Input: part model. Units: mm. Frame: model coordinates. Coordinates: 2 decimals unless noted, no trailing zeros. Loops run counter-clockwise (first coordinate to the right, second up) from the corner with the lowest first, then second, coordinate; pieces in that order, holes last.
Item 1: Ray query, line 1 along X through (y, z) = (-72, 0.6); line 2 along Y through (x, z) = (-85, 2.3); line 3 along Y through (x, z) = (0, 1.45). Return the intervals inside material, ascending.
Item 2: Section A-A on y = 59. Return loops of the section in (x, z), and give its area (3 significant figures).
Item 3: Contact query for flat-ended pins moving along their axis: P1, Ø4, axis at x = 50.5, y = -29.5, coming from the -Z side; P2, Ø1.5, axis at x = 92, z = 1.5, coming from the -Y side; P3, Ø2, axis at x = 85, y = -72, coming from the +Z side; P4, Ø1.5, axis at y = -106, z = 1.5, coming from the -X side. Output: stop coordinate, or through.
Item 4: Section B-B on z = 1.2. Give the number of separate pieces and of enclosed holes in the cut face, and give its area (3 significant figures).
Item 5: Pull-direction query (Y, two-part tool) for faces 1 (the cylindrical face through (-1.301, 53.143, 1.521)), 2 (the flat face through (-1, 2, 3)); classes: released by +Y, released by -Y, zero draft, split by the parting line, or undercut.
Autodesk Fusion 360 part; units mm, degrees
sketch "Sketch1" plane through (0, 0, 0) normal (0, 0, 1) x (1, 0, 0)
  line L0 (100, 125) -> (-100, 125)
  line L1 (-100, 125) -> (-100, -125)
  line L2 (-100, -125) -> (100, -125)
  line L3 (100, -125) -> (100, 125)
  line L4 (100, 125) -> (-100, -125) construction
  line L5 (-100, 125) -> (100, -125) construction
  line L6 (-100, 125) -> (100, 125)
  line L7 (100, 125) -> (100, 129)
  line L8 (100, 129) -> (-100, 129)
  line L9 (-100, 129) -> (-100, 125)
  line L10 (-100, -125) -> (100, -125)
  line L11 (100, -125) -> (100, -129)
  line L12 (100, -129) -> (-100, -129)
  line L13 (-100, -129) -> (-100, -125)
  line L14 (100, 125) -> (104, 125)
  line L15 (104, 125) -> (104, -125)
  line L16 (104, -125) -> (100, -125)
  line L17 (100, -125) -> (100, 125)
  line L18 (-100, 125) -> (-104, 125)
  line L19 (-104, 125) -> (-104, -125)
  line L20 (-104, -125) -> (-100, -125)
  line L21 (-100, -125) -> (-100, 125)
  line L22 (-80, -53.8) -> (-80, 2.2) construction
  circle A0 centre (-80, -53.8) radius 1.65 construction
  circle A1 centre (-80, 2.2) radius 1.65 construction
  line L23 (-61.0622, -1) -> (-98.9378, -1) construction
  line L24 (-98.9378, -1) -> (-98.9378, -50.6) construction
  line L25 (-98.9378, -50.6) -> (-61.0622, -50.6) construction
  line L26 (-61.0622, -50.6) -> (-61.0622, -1) construction
  line L27 (-61.0622, -1) -> (-98.9378, -50.6) construction
  line L28 (-98.9378, -1) -> (-61.0622, -50.6) construction
  line L29 (-30.5, 49.5) -> (98.5, 49.5) construction
  line L30 (98.5, 49.5) -> (98.5, -47.5) construction
  line L31 (98.5, -47.5) -> (-30.5, -47.5) construction
  line L32 (-30.5, -47.5) -> (-30.5, 49.5) construction
  circle A2 centre (-28, 43) radius 1.65
  circle A3 centre (94, -42) radius 1.65
  line L33 (-100, 125) -> (-85.5, 125)
  line L34 (-85.5, 125) -> (-85.5, 116)
  line L35 (-85.5, 116) -> (-100, 116)
  line L36 (-100, 116) -> (-100, 125)
  line L37 (100, 125) -> (85.5, 125)
  line L38 (85.5, 125) -> (85.5, 116)
  line L39 (85.5, 116) -> (100, 116)
  line L40 (100, 116) -> (100, 125)
  line L41 (-100, -125) -> (-85.5, -125)
  line L42 (-85.5, -125) -> (-85.5, -116)
  line L43 (-85.5, -116) -> (-100, -116)
  line L44 (-100, -116) -> (-100, -125)
  line L45 (100, -125) -> (85.5, -125)
  line L46 (85.5, -125) -> (85.5, -116)
  line L47 (85.5, -116) -> (100, -116)
  line L48 (100, -116) -> (100, -125)
  line L49 (-100, 100) -> (-104, 100)
  line L50 (100, 100) -> (104, 100)
  line L51 (-100, -100) -> (-104, -100)
  line L52 (100, -100) -> (104, -100)
  line L53 (-85.5, 125) -> (-85.5, 129)
  line L54 (85.5, 125) -> (85.5, 129)
  line L55 (-85.5, -125) -> (-85.5, -129)
  line L56 (85.5, -125) -> (85.5, -129)
  line L57 (-115, -140) -> (-75, -140) construction
  line L58 (-75, -140) -> (-75, -87) construction
  line L59 (-75, -87) -> (-115, -87) construction
  line L60 (-115, -87) -> (-115, -140) construction
  line L61 (-63.3606, -140) -> (-21.3606, -140) construction
  line L62 (-21.3606, -140) -> (-21.3606, -53.8) construction
  line L63 (-21.3606, -53.8) -> (-63.3606, -53.8) construction
  line L64 (-63.3606, -53.8) -> (-63.3606, -140) construction
  line L65 (-100, 0) -> (-118.2487, 0) construction
  circle A4 centre (0, 0) radius 152.5
  circle A5 centre (-85, -72) radius 1.65
  line L66 (-85, -72) -> (85, -72) construction
  line L67 (85, -72) -> (85, 72) construction
  line L68 (85, 72) -> (-85, 72) construction
  line L69 (-85, 72) -> (-85, -72) construction
  circle A6 centre (85, 72) radius 1.65
  circle A7 centre (85, -72) radius 1.65
  circle A8 centre (-85, 72) radius 1.65
  point P0 (-80, -25.8)
  dimension "d1" = 200
  dimension "d2" = 250
  dimension "d3" = 4
  dimension "d4" = 4
  dimension "d5" = 4
  dimension "d6" = 4
  dimension "d7" = 20
  dimension "d8" = 56
  dimension "d10" = 3.3
  dimension "d11" = 37.8755
  dimension "d12" = 49.6
  dimension "d13" = 2.5
  dimension "d14" = 6.5
  dimension "d15" = 3.3
  dimension "d16" = 5.5
  dimension "d17" = 4.5
  dimension "d18" = 129
  dimension "d19" = 97
  dimension "d20" = 1.5
  dimension "d21" = 14.5
  dimension "d22" = 9
  dimension "d23" = 14.5
  dimension "d24" = 9
  dimension "d25" = 14.5
  dimension "d26" = 14.5
  dimension "d27" = 9
  dimension "d28" = 9
  dimension "d29" = 25
  dimension "d30" = 25
  dimension "d31" = 25
  dimension "d32" = 25
  dimension "d33" = 40
  dimension "d34" = 53
  dimension "d35" = 15
  dimension "d36" = 15
  dimension "d37" = 3.3
  dimension "d38" = 86.2
  dimension "d39" = 42
  dimension "d40" = 1
  dimension "d50" = 305
  dimension "d51" = 3.3
  dimension "d52" = 15
  dimension "d53" = 15
  dimension "d54" = 15
  dimension "d55" = 53
  dimension "d56" = 53
  dimension "d57" = 170
  dimension "d58" = 144
  dimension "d60" = 47.5
  dimension "d61" = 49.5
extrude "Extrude1" add sketch "Sketch1" along normal blind 3 contours L0 L1 L2 L3 L6 L10 L17 L21 L34 L35 L38 L39 L42 L43 L46 L47 A4 | L0 L6 L8 L53 L54 A4 | L3 L15 L17 L50 L52 | L1 L19 L21 L49 L51 | L2 L10 L12 L55 L56 A4
sketch "Sketch2" plane through (0, 0, 3) normal (0, 0, 1) x (1, 0, 0)
  circle A0 centre (85, -72) radius 1.65
  circle A1 centre (-85, -72) radius 1.65
  circle A2 centre (85, 72) radius 1.65
  circle A3 centre (94, -42) radius 1.65
  circle A4 centre (-85, 72) radius 1.65
  circle A5 centre (-28, 43) radius 1.65
  line L0 (100, 100) -> (100, 115.1358)
  arc A6 (100, 115.1358) -> (98.9962, 116) centre (0, 0) ccw
  line L1 (98.9962, 116) -> (85.5, 116)
  line L2 (85.5, 116) -> (85.5, 126.2775)
  arc A7 (85.5, 126.2775) -> (81.3342, 129) centre (0, 0) ccw
  line L3 (81.3342, 129) -> (-81.3342, 129)
  arc A8 (-81.3342, 129) -> (-85.5, 126.2775) centre (0, 0) ccw
  line L4 (-85.5, 126.2775) -> (-85.5, 116)
  line L5 (-85.5, 116) -> (-98.9962, 116)
  arc A9 (-98.9962, 116) -> (-100, 115.1358) centre (0, 0) ccw
  line L6 (-100, 115.1358) -> (-100, 100)
  line L7 (-100, 100) -> (-104, 100)
  line L8 (-104, 100) -> (-104, -100)
  line L9 (-104, -100) -> (-100, -100)
  line L10 (-100, -100) -> (-100, -115.1358)
  arc A10 (-100, -115.1358) -> (-98.9962, -116) centre (0, 0) ccw
  line L11 (-98.9962, -116) -> (-85.5, -116)
  line L12 (-85.5, -116) -> (-85.5, -126.2775)
  arc A11 (-85.5, -126.2775) -> (-81.3342, -129) centre (0, 0) ccw
  line L13 (-81.3342, -129) -> (81.3342, -129)
  arc A12 (81.3342, -129) -> (85.5, -126.2775) centre (0, 0) ccw
  line L14 (85.5, -126.2775) -> (85.5, -116)
  line L15 (85.5, -116) -> (98.9962, -116)
  arc A13 (98.9962, -116) -> (100, -115.1358) centre (0, 0) ccw
  line L16 (100, -115.1358) -> (100, -100)
  line L17 (100, -100) -> (104, -100)
  line L18 (104, -100) -> (104, 100)
  line L19 (104, 100) -> (100, 100)
  line L20 (-10, 129) -> (10, 129)
  line L21 (10, 129) -> (10, 111)
  line L22 (8, 109) -> (-8, 109)
  line L23 (-10, 111) -> (-10, 129)
  arc A14 (-10, 111) -> (-8, 109) centre (-8, 111) ccw
  arc A15 (8, 109) -> (10, 111) centre (8, 111) ccw
  point P0 (10, 109)
  point P1 (-10, 109)
  dimension "d62" = 20
  dimension "d63" = 20
  dimension "d64" = 2
extrude "Extrude2" cut sketch "Sketch2" against normal blind 3 contours L3 L20 L21 L22 L23 A14 A15
fillet "Fillet4" radius 2 2 edges at (-10, 129, 1.5) (10, 129, 1.5)
sketch "Sketch3" plane through (0, 0, 3) normal (0, 0, 1) x (1, 0, 0)
  arc A0 (12, 129) -> (10, 127) centre (12, 127) ccw
  line L0 (10, 127) -> (10, 111)
  arc A1 (8, 109) -> (10, 111) centre (8, 111) ccw
  line L1 (8, 109) -> (-8, 109)
  arc A2 (-10, 111) -> (-8, 109) centre (-8, 111) ccw
  line L2 (-10, 111) -> (-10, 127)
  arc A3 (-10, 127) -> (-12, 129) centre (-12, 127) ccw
  line L3 (-12, 129) -> (-81.3342, 129)
  arc A4 (-81.3342, 129) -> (-85.5, 126.2775) centre (0, 0) ccw
  line L4 (-85.5, 126.2775) -> (-85.5, 116)
  line L5 (-85.5, 116) -> (-98.9962, 116)
  arc A5 (-98.9962, 116) -> (-100, 115.1358) centre (0, 0) ccw
  line L6 (-100, 115.1358) -> (-100, 100)
  line L7 (-100, 100) -> (-104, 100)
  line L8 (-104, 100) -> (-104, -100)
  line L9 (-104, -100) -> (-100, -100)
  line L10 (-100, -100) -> (-100, -115.1358)
  arc A6 (-100, -115.1358) -> (-98.9962, -116) centre (0, 0) ccw
  line L11 (-98.9962, -116) -> (-85.5, -116)
  line L12 (-85.5, -116) -> (-85.5, -126.2775)
  arc A7 (-85.5, -126.2775) -> (-81.3342, -129) centre (0, 0) ccw
  line L13 (-81.3342, -129) -> (81.3342, -129)
  arc A8 (81.3342, -129) -> (85.5, -126.2775) centre (0, 0) ccw
  line L14 (85.5, -126.2775) -> (85.5, -116)
  line L15 (85.5, -116) -> (98.9962, -116)
  arc A9 (98.9962, -116) -> (100, -115.1358) centre (0, 0) ccw
  line L16 (100, -115.1358) -> (100, -100)
  line L17 (100, -100) -> (104, -100)
  line L18 (104, -100) -> (104, 100)
  line L19 (104, 100) -> (100, 100)
  line L20 (100, 100) -> (100, 115.1358)
  arc A10 (100, 115.1358) -> (98.9962, 116) centre (0, 0) ccw
  line L21 (98.9962, 116) -> (85.5, 116)
  line L22 (85.5, 116) -> (85.5, 126.2775)
  arc A11 (85.5, 126.2775) -> (81.3342, 129) centre (0, 0) ccw
  line L23 (81.3342, 129) -> (12, 129)
  circle A12 centre (85, -72) radius 1.65
  circle A13 centre (-85, -72) radius 1.65
  circle A14 centre (85, 72) radius 1.65
  circle A15 centre (94, -42) radius 1.65
  circle A16 centre (-85, 72) radius 1.65
  circle A17 centre (-28, 43) radius 1.65
  circle A18 centre (0, 59) radius 6
  dimension "d69" = 12
  dimension "d70" = 50
  dimension "d71" = 104
extrude "Extrude3" cut sketch "Sketch3" against normal blind 3 contours A18
sketch "Sketch4" plane through (0, 0, 3) normal (0, 0, 1) x (1, 0, 0)
  circle A0 centre (0, 59) radius 6
  arc A1 (12, 129) -> (10, 127) centre (12, 127) ccw
  line L0 (10, 127) -> (10, 111)
  arc A2 (8, 109) -> (10, 111) centre (8, 111) ccw
  line L1 (8, 109) -> (-8, 109)
  arc A3 (-10, 111) -> (-8, 109) centre (-8, 111) ccw
  line L2 (-10, 111) -> (-10, 127)
  arc A4 (-10, 127) -> (-12, 129) centre (-12, 127) ccw
  line L3 (-12, 129) -> (-81.3342, 129)
  arc A5 (-81.3342, 129) -> (-85.5, 126.2775) centre (0, 0) ccw
  line L4 (-85.5, 126.2775) -> (-85.5, 116)
  line L5 (-85.5, 116) -> (-98.9962, 116)
  arc A6 (-98.9962, 116) -> (-100, 115.1358) centre (0, 0) ccw
  line L6 (-100, 115.1358) -> (-100, 100)
  line L7 (-100, 100) -> (-104, 100)
  line L8 (-104, 100) -> (-104, -100)
  line L9 (-104, -100) -> (-100, -100)
  line L10 (-100, -100) -> (-100, -115.1358)
  arc A7 (-100, -115.1358) -> (-98.9962, -116) centre (0, 0) ccw
  line L11 (-98.9962, -116) -> (-85.5, -116)
  line L12 (-85.5, -116) -> (-85.5, -126.2775)
  arc A8 (-85.5, -126.2775) -> (-81.3342, -129) centre (0, 0) ccw
  line L13 (-81.3342, -129) -> (81.3342, -129)
  arc A9 (81.3342, -129) -> (85.5, -126.2775) centre (0, 0) ccw
  line L14 (85.5, -126.2775) -> (85.5, -116)
  line L15 (85.5, -116) -> (98.9962, -116)
  arc A10 (98.9962, -116) -> (100, -115.1358) centre (0, 0) ccw
  line L16 (100, -115.1358) -> (100, -100)
  line L17 (100, -100) -> (104, -100)
  line L18 (104, -100) -> (104, 100)
  line L19 (104, 100) -> (100, 100)
  line L20 (100, 100) -> (100, 115.1358)
  arc A11 (100, 115.1358) -> (98.9962, 116) centre (0, 0) ccw
  line L21 (98.9962, 116) -> (85.5, 116)
  line L22 (85.5, 116) -> (85.5, 126.2775)
  arc A12 (85.5, 126.2775) -> (81.3342, 129) centre (0, 0) ccw
  line L23 (81.3342, 129) -> (12, 129)
  circle A13 centre (85, -72) radius 1.65
  circle A14 centre (-85, -72) radius 1.65
  circle A15 centre (85, 72) radius 1.65
  circle A16 centre (94, -42) radius 1.65
  circle A17 centre (-85, 72) radius 1.65
  circle A18 centre (-28, 43) radius 1.65
equation "d4 = d3"
equation "d5 = d3"
equation "d6 = d3"
equation "d23 = d21"
equation "d24 = d22"
equation "d25 = d21"
equation "d26 = d25"
equation "d27 = d22"
equation "d28 = d24"
equation "d30 = d29"
equation "d31 = d29"
equation "d32 = d29"
equation "d36 = d35"
equation "d60 = d19 / 2 - 1 mm"
Results found:
1. line 1: x = -104 to -86.65, -83.35 to 83.35, 86.65 to 104
1. line 2: y = -126.61 to -73.65, -70.35 to 70.35, 73.65 to 126.61
1. line 3: y = -129 to 53, 65 to 109
2. outline: (-104, 0) - (-6, 0) - (-6, 3) - (-104, 3) - close; (6, 0) - (104, 0) - (104, 3) - (6, 3) - close
2. area: 588 mm2
3. P1: stops at z = 0
3. P2: stops at y = -116
3. P3: passes through
3. P4: stops at x = -100
4. separate pieces: 1
4. enclosed holes: 7
4. area: 51,900 mm2
5. face 1: undercut
5. face 2: zero draft
